Geometry: final body of the model. Coordinates: model frame, mm. A direction names the side the tool comes from. Give positions to 0.01 mm unless a question says otherwise; leave off trailing zeros. Write each loop counter-clockwise with the first axis right and the second up, starting at its lowest first coordinate (ties: lowest second). Pieces come first, ordered by that corner, then holes. Notation, with made-up numbers: (63, 19) -> (115, 19) arc R12 ccw to (115, 38) -> close; hole circle Ø9 at (4.25, -0.5). An arc over 180 degrees is marked (long way). Answer as a JSON object with one key per item and string values.
Autodesk Inventor part; units mm, degrees
ref_plane "YZ Plane" through (0, 0, 0) normal (1, 0, 0) x (0, 1, 0)
ref_plane "XZ Plane" through (0, 0, 0) normal (0, 1, 0) x (-1, 0, 0)
ref_plane "XY Plane" through (0, 0, 0) normal (0, 0, 1) x (1, 0, 0)
sketch "Sketch1" plane through (0, 0, 0) normal (0, 0, 1) x (1, 0, 0)
  line L0 (0, 0) -> (0, 50)
  line L1 (0, 50) -> (18, 50)
  line L2 (18, 50) -> (18, 30)
  line L3 (18, 30) -> (5, 30)
  line L4 (5, 30) -> (5, 0)
  line L5 (5, 0) -> (0, 0)
  dimension "d0" = 50
  dimension "d1" = 18
  dimension "d2" = 20
  dimension "d3" = 13
revolve "Revolution1" add sketch "Sketch1" angle 360 about axis through (0, 0, 0) along (0, 1, 0)
sketch "Sketch2" plane through (0, 50, 0) normal (0, 1, 0) x (1, 0, 0)
  circle A0 centre (0, 0) radius 18
  circle A1 centre (0, 0) radius 13
  dimension "d5" = 5
extrude "Extrusion1" cut sketch "Sketch2" against normal blind 15 contours A1
sketch "Sketch3" plane through (0, 0, 0) normal (0, 0, 1) x (1, 0, 0)
  line L0 (5, 0) -> (-5, 0)
  line L1 (5, 12) -> (-5, 12)
  line L2 (5, 12) -> (4, 12)
  line L3 (4, 12) -> (4, 0)
  line L4 (4, 0) -> (5, 0)
  line L5 (5, 0) -> (5, 12)
  point P0 (0, 0)
  dimension "d8" = 12
extrude "Extrusion2" cut sketch "Sketch3" along normal through all both and the other way through all
sketch "Sketch4" plane through (0, 0, 0) normal (0, 0, 1) x (1, 0, 0)
  line L0 (4, 0) -> (-5, 0)
  circle A0 centre (0, 6) radius 2
  point P0 (0, 0)
  dimension "d11" = 6
  dimension "d12" = 4
extrude "Extrusion3" cut sketch "Sketch4" along normal through all both and the other way through all
properties part number "shellerAdapter" material "Stainless Steel, Austenitic"
Q1. Material intervals for L1, parallel to Z at x = 0, y = 39.5; L2, parallel to Y at x = 0, z = 2.25, sorted ascending. Write a range as from..to.
Values:
{"L1": "-18..-13, 13..18", "L2": "0..4, 8..35"}
Q2. Cut plane B-B (x = 0). Return the cut outline in (y, z), and give its area (3 significant figures).
Values:
{"outline": "(0, -5) -> (4, -5) -> (4, 5) -> (0, 5) -> close; (8, -5) -> (30, -5) -> (30, -18) -> (50, -18) -> (50, -13) -> (35, -13) -> (35, 13) -> (50, 13) -> (50, 18) -> (30, 18) -> (30, 5) -> (8, 5) -> close", "area": "590 mm²"}
Q3. Cut plane D-D (x = 10). Return the cut outline in (y, z).
Values:
{"outline": "(30, -14.97) -> (50, -14.97) -> (50, -8.31) -> (35, -8.31) -> (35, 8.31) -> (50, 8.31) -> (50, 14.97) -> (30, 14.97) -> close"}
Q4. Mould query, pull axis Y, two halves, no side actions, for faces 4 (the cylindrical face through (-2.343, 39.86, 17.847)), 5 (the cylindrical face through (0, 8, 0)), 6 (the flat face through (4, 30, 4)). Classes: pulls with the +Y half, pulls with the -Y half, needs draft (parallel to the pull), parting line crosses it, or undercut.
Values:
{"face 4": "needs draft", "face 5": "undercut", "face 6": "pulls with the -Y half"}
Q5. Set-up query: faces 1 (the flat face through (4, 6, 0)), 2 (the cylindrical face through (-5, 15, 0)), 3 (the flat face through (0, 35, 0)). Return all of +Z, -Z, +X, -X, +Y, -Y with unobstructed straight access to the full face (end or side cutting, diameter ignored); none if empty.
Values:
{"face 1": "+Z, -Z, +X, -Y", "face 2": "-Y", "face 3": "+Y"}
Q6. Cut plane A-A (z = 0). Return the cut outline in (x, y).
Values:
{"outline": "(-18, 30) -> (-5, 30) -> (-5, 0) -> (4, 0) -> (4, 12) -> (5, 12) -> (5, 30) -> (18, 30) -> (18, 50) -> (13, 50) -> (13, 35) -> (-13, 35) -> (-13, 50) -> (-18, 50) -> close; hole circle Ø4 at (0, 6)"}
Q7. Cut plane C-C (y = 45). Return the cut outline in (x, z), and give its area (3 significant figures).
Values:
{"outline": "circle Ø36 at (0, 0); hole circle Ø26 at (0, 0)", "area": "487 mm²"}
Q8. First-contact query: P1, Ø0.8, axis at x = 4.5, z = 0, coming from the -Y side; P2, Ø8, axis at x = -1.5, z = 4.5, coming from the +Y side; P3, Ø2, axis at x = 2, y = 21.5, coming from the +Z side. Flat tips, straight axial feed; report the tip coordinate or a pass-through.
Values:
{"P1": "y = 12", "P2": "y = 35", "P3": "z = 4.9"}
